Design review of the part shown in the three views and the two pictorial views. Dimensions are in mm from the part's minimum x, y and z. Round coordinates to 2 decimals unless told otherwise and drop trailing zeros. Write each loop counter-clockwise with the first axis right and the second up, starting at its lowest first coordinate (ties: lowest second). Pieces come first, ordered by that corner, then holes. Notation, with made-up numbers: (25.25, 60.25) -> (49.25, 60.25) arc R17 cw to (49.25, 86.25) -> close; hole circle Ø4 at (12.25, 36.5). An arc over 180 degrees is marked (long way). Return JSON: item names as keys, results as strings. Group by question number.
1. Take a section at D-D, the plane x = 50. Write out the cut boundary in (y, z).
2. Take a section at A-A, the plane y = 4. Write out the cut boundary in (x, z).
3. Take a section at B-B, the plane y = 28. Give the number of separate pieces and of enclosed holes in the cut face, then the cut area to 3 significant figures.
4. For line 1 along Y through (x, z) = (97, 4.9); line 2 along Y through (x, z) = (3, 1); line 3 along X through (y, z) = (30, 4.9) (1 decimal), list the stretches that pass through material, from the lowest coordinate up. Write a range as from..to.
5. Clearance check with flat-ended pins moving along their axes: P1, Ø1.9, axis at x = 3.5, y = 11, coming from the +Z side; P2, Ø3, axis at x = 97, y = 28, coming from the +Z side. State where each tip first meets the part, or that it passes through.
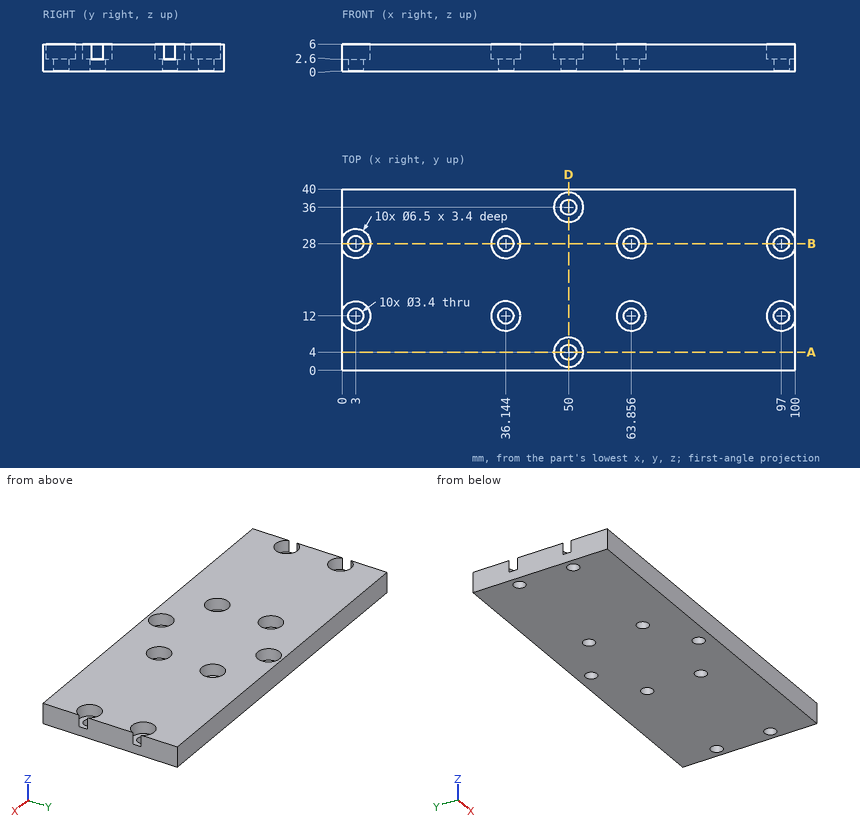
Output:
{
 "1": {"outline": "(0, 0) -> (2.3, 0) -> (2.3, 2.6) -> (0.75, 2.6) -> (0.75, 6) -> (0, 6) -> close; (5.7, 0) -> (34.3, 0) -> (34.3, 2.6) -> (32.75, 2.6) -> (32.75, 6) -> (7.25, 6) -> (7.25, 2.6) -> (5.7, 2.6) -> close; (37.7, 0) -> (40, 0) -> (40, 6) -> (39.25, 6) -> (39.25, 2.6) -> (37.7, 2.6) -> close"},
 "2": {"outline": "(0, 0) -> (48.3, 0) -> (48.3, 2.6) -> (46.75, 2.6) -> (46.75, 6) -> (0, 6) -> close; (51.7, 0) -> (100, 0) -> (100, 6) -> (53.25, 6) -> (53.25, 2.6) -> (51.7, 2.6) -> close"},
 "3": {"separate pieces": "5", "enclosed holes": "0", "area": "478 mm^2"},
 "4": {"line 1": "y = 0..8.75, 15.25..24.75, 31.25..40", "line 2": "y = 0..10.3, 13.7..26.3, 29.7..40", "line 3": "x = 0..0.4, 5.6..33.6, 38.7..61.3, 66.4..94.4, 99.6..100"},
 "5": {"P1": "stops at z = 2.6", "P2": "passes through"}
}
